Input: dimensioned drawing with shaded views. Units: mm. Origin: part minimum x, y, z. A direction names the side the tool comes from. Round coordinates to 2 decimals unless told otherwise and drop trailing zeros. Write each loop counter-clockwise with the first axis right and the second up, starting at its lowest first coordinate (ties: lowest second). Pieces come first, ordered by that corner, then holes. Notation, with made-up numbers: M 55,17 L 68,17 A7 ccw 68,22 Z; hole C -15.75,65.25 d6. An arc over 180 degrees is marked long. Use one line per item in the form item = value. Start each with the question number.
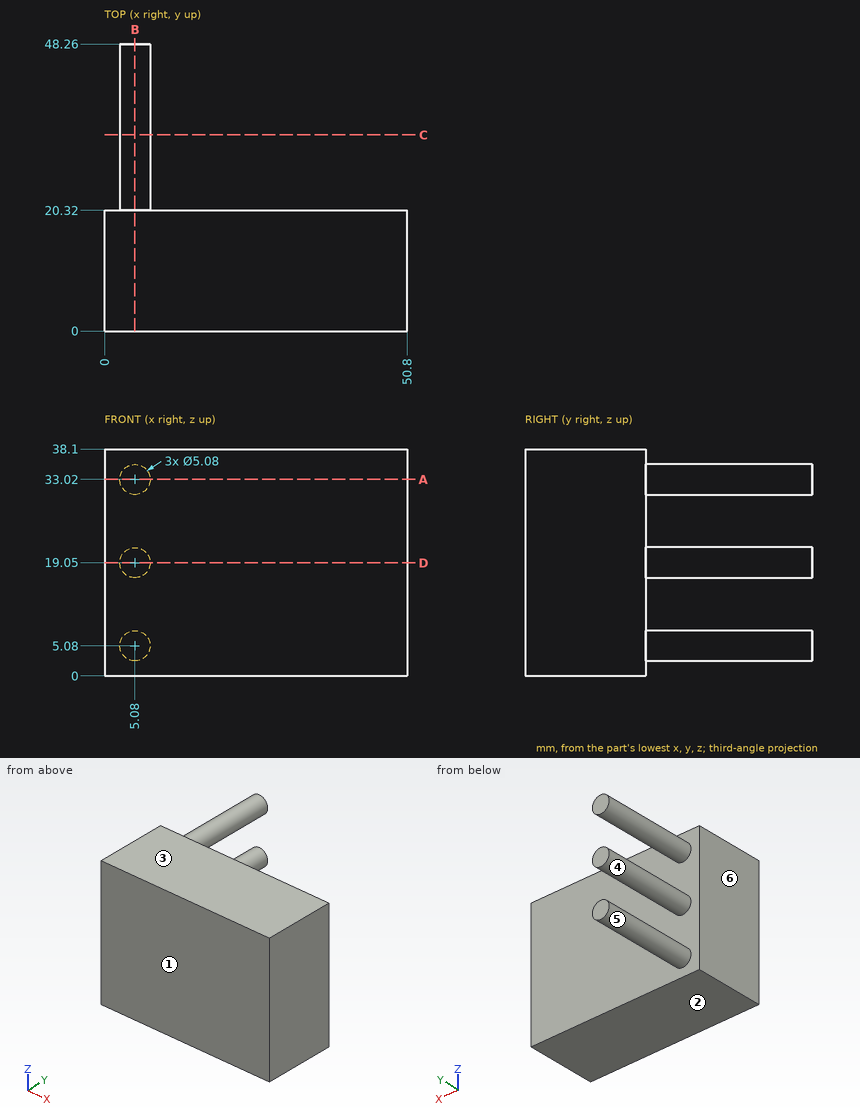
1. Pull-direction query (Z, two-part tool) for the marked faces 1, 2, 3 and 4; classes: released by +Z, released by -Z, zero draft, split by the parting line, or undercut.
2. Section query B-B (x = 5.08). Return loops of the section in (y, z).
3. Section query A-A (z = 33.02). Return loops of the section in (x, y), then the cut area to 3 significant figures.
4. Ray query, probe 1 along Y at (x, z) = (48.5, 12); probe 2 along X at (y, z) = (44.5, 5); probe 3 along X at (y, z) = (30.5, 33.5). Return the intervals inside material, ascending.
5. Contact query for flat-ended pins moving along their axis: pin 1 (1.5 mm diameter, centred on x = 24, z = 33, fed in from +Y); pin 2 (1 mm diameter, centred on y = 23, z = 8.5, fed in from -X); pin 3 (12 mm diameter, centred on x = 10.5, y = 31, fed in from +Z). Output: stop coordinate, or through.
6. Set-up query: the marked faces 5 and 6. Return all of +Z, -Z, +X, -X, +Y, -Y with unobstructed straight access to the full face (end or side cutting, diameter ignored); none if empty.
7. Section query C-C (y = 33). Return loops of the section in (x, z).
Checks:
q1.face_1 = zero draft
q1.face_2 = released by -Z
q1.face_3 = released by +Z
q1.face_4 = undercut
q2.outline = M 0,0 L 20.32,0 L 20.32,2.54 L 48.26,2.54 L 48.26,7.62 L 20.32,7.62 L 20.32,16.51 L 48.26,16.51 L 48.26,21.59 L 20.32,21.59 L 20.32,30.48 L 48.26,30.48 L 48.26,35.56 L 20.32,35.56 L 20.32,38.1 L 0,38.1 Z
q3.outline = M 0,0 L 50.8,0 L 50.8,20.32 L 7.62,20.32 L 7.62,48.26 L 2.54,48.26 L 2.54,20.32 L 0,20.32 Z
q3.area = 1,170 mm^2
q4.probe_1 = 0 to 20.32
q4.probe_2 = 2.54 to 7.62
q4.probe_3 = 2.59 to 7.57
q5.pin_1 = 20.32
q5.pin_2 = through
q5.pin_3 = 35.56
q6.face_5 = +Y
q6.face_6 = +Z, -Z, -X, +Y, -Y
q7.outline = C 5.08,5.08 d5.08; C 5.08,19.05 d5.08; C 5.08,33.02 d5.08
